Design review of the part shown in the three views and the two pictorial views. Dimensions are in mm from the part's minimum x, y and z. A direction names the side the tool comes from. Coordinates: 2 decimals unless noted, no trailing zeros. Write each loop counter-clockwise with the first axis right and the second up, starting at its lowest first coordinate (ties: lowest second). Pieces come first, ordered by that corner, then holes.
Q1. Take a section at B-B, the plane z = 24.5. Write out the cut boundary in (x, y), plus the area to 3 significant figures.
Q2. Take a section at D-D, the plane y = 7. Write out the cut boundary in (x, z).
Q3. For L1, parallel to Y at x = 26.5, z = 34; L2, parallel to X at y = 18.5, z = 23.5; L3, parallel to Z at x = 34, y = 38.5, list the stretches that pass through material, from the lowest coordinate up.
Q4. Take a section at A-A, the plane y = 17. Write out the cut boundary in (x, z), plus the area to 3 significant figures.
Q5. For the marked faces 1 and 2, list the 3-axis set-ups (+Z, -Z, +X, -X, +Y, -Y) from which the entire face can be reached by the end or side of a thin tool; tool diameter is ignored.
Q6. For pin 1 Ø2 at (x, z) = (36.5, 13.5) entering from -Y; pin 2 Ø1.5 at (x, z) = (61.5, 17.5) entering from -Y; pin 3 Ø12 at (x, y) = (44.5, 26.5) entering from +Z, all flat-tipped, find the tip position at first contact; note any pin that passes through.
Q7. Take a section at C-C, the plane x = 9. Write out the cut boundary in (y, z).
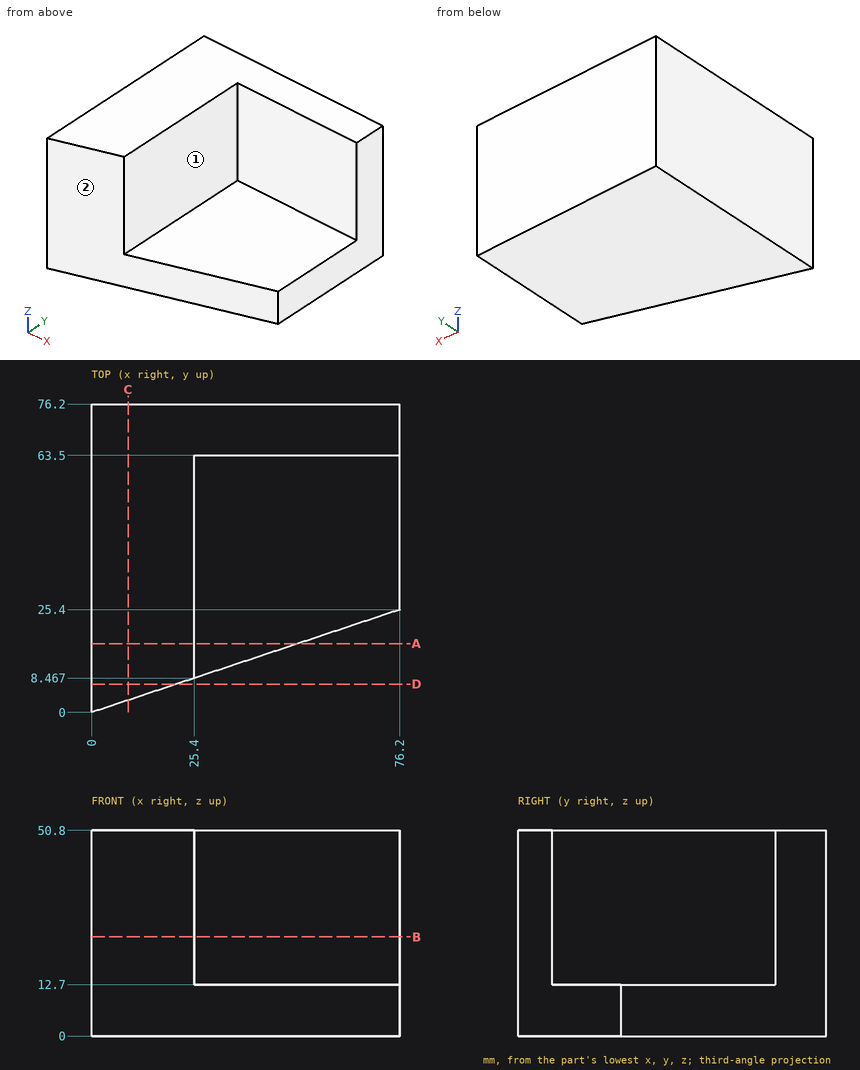
Responses:
1. outline: (0, 0) - (25.4, 8.47) - (25.4, 63.5) - (76.2, 63.5) - (76.2, 76.2) - (0, 76.2) - close
1. area: 2,470 mm2
2. outline: (0, 0) - (21, 0) - (21, 50.8) - (0, 50.8) - close
3. L1: y = 63.5 to 76.2
3. L2: x = 0 to 25.4
3. L3: z = 0 to 12.7
4. outline: (0, 0) - (51, 0) - (51, 12.7) - (25.4, 12.7) - (25.4, 50.8) - (0, 50.8) - close
4. area: 1,620 mm2
5. face 1: +Z, +X, -Y
5. face 2: +Z, -Z, +X, -Y
6. pin 1: stops at y = 11.97
6. pin 2: stops at y = 63.5
6. pin 3: stops at z = 12.7
7. outline: (3, 0) - (76.2, 0) - (76.2, 50.8) - (3, 50.8) - close
